For this review, take the finished solid that the model builds, in its own axes (mm). A direction names the side the tool comes from. Give positions to 0.01 mm unless a question says otherwise; leave off trailing zeros.
Item 1: Consider section A-A (y = -33.5). Give the number of separate pieces and of enclosed holes in the cut face, plus the area to 3 significant figures.
Item 2: The part is to be moulded in two halves that separate along X. For faces 6 (the flat face through (-5, -32, 1)), 7 (the flat face through (0, -32, -3)), 8 (the cylindrical face through (-44.83, -14.12, -2.21)), say which applies: released by +X, released by -X, zero draft, split by the parting line, or undercut.
Item 3: For probe 1 along X at (y, z) = (-35, -1.75); probe 2 along X at (y, z) = (-36, 2.5); probe 3 along Y at (x, z) = (6, 0.75), list the stretches that pass through material, from the lowest coordinate up.
Item 4: Machinability: for faces 1 (the cylindrical face through (-4.19, -26.6, -2.43)), 2 (the flat face through (-0.5, -46, 4)), 3 (the cylindrical face through (4.211, -27.674, 1.981)), 4 (the cylindrical face through (5.74, -39.92, 1.06)), 5 (the flat face through (-3.4, -31, 2)), which of the approach directions +Z, -Z, +X, -X, +Y, -Y give a long, thin tool a straight path to every point of the face, cutting with its end or side? Answer none if there is none.
Item 5: For P1, Ø1.5, axis at y = -11.5, z = 2, coming from the -X side; P2, Ø0.5, axis at x = 0, z = 4, coming from the -Y side; P3, Ø1.8, axis at x = 4, z = 0, coming from the +Y side; P4, Ø12, axis at x = 33.5, y = -33, coming from the -Z side, all flat-tipped, find the tip position at first contact; note any pin that passes through.
```python
from build123d import *

# Parameters (mm, degrees)
F2_R      = 2.4
F3_R      = 2.39999
F5_W      = 10
F5_H      = 8
F7_R      = 1.6
F8_DEPTH  = 5
F7_W      = 4.6828329376
F7_H      = 1.903038422
F9_DEPTH  = 3.4
F10_R     = 2
F11_W     = 4
F11_H     = 4
F12_DEPTH = 0.5


# Not quite as in the source:
# - a fillet or chamfer is up to 0.001 mm smaller than in the source, because OpenCascade refuses the exact size
# - a feature names something its author has since deleted; it is built from what else it names


with BuildPart() as f1:
    # F0 (on Front) → F1 (revolve)
    with BuildSketch(Plane.XZ):
        Polygon((-41, 5), (-47, 5), (-47, 3.4), (-43, 3.4), (-43, -1.4), (-47, -1.4), (-47, -3), (-41, -3), align=None)
    revolve(axis=Axis((0, 0, 0.7178727537), (0, 0, 1)))

    # F2
    f2_edges = [f1.edges().sort_by_distance(p)[0] for p in [
        (43, 0, 3.4),
    ]]
    fillet(f2_edges, radius=F2_R)

    # F3 (radius 2.4 in the source; OpenCascade refuses exactly that, so slightly less here)
    f3_edges = [f1.edges().sort_by_distance(p)[0] for p in [
        (43, 0, -1.4),
    ]]
    fillet(f3_edges, radius=F3_R)

    # F5 (on offset) → F6 (join, up to the next surface of F1)
    with BuildSketch(Plane.XZ.offset(26)):
        with Locations((0, 1)):
            Rectangle(F5_W, F5_H)
    extrude(until=Until.NEXT)

    # F7 (on Right) → F8 (cut, symmetric)
    with BuildSketch(Plane.YZ):
        with Locations((-29.2, 1.5)):
            Circle(F7_R)
    extrude(amount=F8_DEPTH, both=True, mode=Mode.SUBTRACT)

    # F7 (on Right) → F9 (cut, symmetric)
    with BuildSketch(Plane.YZ):
        Polygon((-26, 5.4147794951), (-36.4011118985, 5.4147794951), (-30.6828329376, -1.4), (-26, -1.4), (-26, 3.0355471618), align=None)
        with Locations((-29.2, 1.5)):
            Circle(F7_R, mode=Mode.SUBTRACT)
        with Locations((-28.3414164688, -2.351519211)):
            Rectangle(F7_W, F7_H)
    extrude(amount=F9_DEPTH, both=True, mode=Mode.SUBTRACT)

    # F10
    f10_edges = [f1.edges().sort_by_distance(p)[0] for p in [
        (-4.2, -26, 5),
        (4.2, -26, 5),
        (-4.2, -26, -3),
        (4.2, -26, -3),
        (-5, -40.69398, 1),
        (5, -40.69398, 1),
    ]]
    fillet(f10_edges, radius=F10_R)

    # F11 (on Right) → F12 (cut, symmetric)
    with BuildSketch(Plane.YZ):
        with Locations((-46, 3)):
            Rectangle(F11_W, F11_H)
    extrude(amount=F12_DEPTH, both=True, mode=Mode.SUBTRACT)


solid = f1.part
```
Resolved:
1. separate pieces: 3
1. enclosed holes: 0
1. area: 159 mm2
2. face 6: undercut
2. face 7: zero draft
2. face 8: split by the parting line
3. probe 1: x = -31.37 to -21.35, -5 to 5, 21.35 to 31.37
3. probe 2: x = -24.47 to -19.62, -5 to 5, 19.62 to 24.47
3. probe 3: y = -42.59 to -40.1, 40.56 to 42.59
4. face 1: -Z
4. face 2: +Z, -Y
4. face 3: none
4. face 4: +Z, -Z
4. face 5: +Z
5. P1: stops at x = -42.24
5. P2: stops at y = -44
5. P3: stops at y = 43.75
5. P4: stops at z = -3
